```python
from build123d import *

# Parameters (mm, degrees)
F0_W     = 60
F0_H     = 43
F0_R     = 6
F1_DEPTH = 34


with BuildPart() as f1:
    # F0 (on Front) → F1 (new body)
    with BuildSketch(Plane.XZ):
        Rectangle(F0_W, F0_H)
        with Locations((0, 3.5)):
            Circle(F0_R, mode=Mode.SUBTRACT)
    extrude(amount=-F1_DEPTH)


solid = f1.part
```
Can you work these out from the model? Positions are in its coordinate system, mm. Round coordinates to 2 decimals unless told otherwise and drop trailing zeros. Order: outer loops, then holes, each group sorted by start corner. A loop starts at its lowest first (then second) coordinate and runs counter-clockwise, first axis right, second up.
(1) If I drill on L1, parallel to Z at x = 0, y = 17; L2, parallel to Z at x = -5.5, y = 31.5; L3, parallel to X at y = 11, z = 3, over which ranges is the centre line in solid material (lowest first)?
Results are:
L1: z = -21.5 to -2.5, 9.5 to 21.5
L2: z = -21.5 to 1.1, 5.9 to 21.5
L3: x = -30 to -5.98, 5.98 to 30
(2) If we section it at B-B (x = 0): Please give me the cut outline in (y, z).
Results are:
outline: (0, -21.5) - (34, -21.5) - (34, -2.5) - (0, -2.5) - close; (0, 9.5) - (34, 9.5) - (34, 21.5) - (0, 21.5) - close
(3) We'd pull the mould along X, two halves only. Please class faces 1 (the face through (-30, 17, 0)), 2 (the face through (-5.994, 16.762, 3.764)), 3 (the face through (30, 17, 0)), 4 (the face through (0, 34, -4)): +X half, -X half, draft (parallel to the pull), parting line (faces both ways), or undercut.
Results are:
face 1: -X half
face 2: undercut
face 3: +X half
face 4: draft
(4) If we section it at A-A (z = 3.5): Please give me the cut outline in (x, y), plus the area to 3 significant figures.
Results are:
outline: (-30, 0) - (-6, 0) - (-6, 34) - (-30, 34) - close; (6, 0) - (30, 0) - (30, 34) - (6, 34) - close
area: 1,630 mm2
(5) If we section it at C-C (y = 27): Please give me the cut outline in (x, z).
Results are:
outline: (-30, -21.5) - (30, -21.5) - (30, 21.5) - (-30, 21.5) - close; hole circle Ø12 at (0, 3.5)
